Source: CAD feature listing. Evaluate the final solid. Frame: model axes, mm. Round coordinates to 2 decimals unless told otherwise and drop trailing zeros. Loops run counter-clockwise (first coordinate to the right, second up) from the corner with the lowest first, then second, coordinate; pieces in that order, holes last. Notation, with made-up numbers: (41, 54) -> (99, 54) arc R20 ccw to (99, 65) -> close; hole circle Ø3 at (47, 19.25). An arc over 180 degrees is marked (long way). Put each result on its own line as item: value. Start each with the question number.
1. Cut plane B-B (y = -195). Return the cut outline in (x, z) (3 decimals).
2. Cut plane D-D (y = 94.5). Return the cut outline in (x, z) (3 decimals), then the cut area to 3 significant figures.
3. Cut plane C-C (x = 47). Return the cut outline in (y, z) (3 decimals).
4. Contact query for flat-ended pins moving along their axis: pin 1 (3 mm diameter, centred on y = -86.5, z = 1, fed in from -X); pin 2 (3 mm diameter, centred on x = 89.5, z = 2, fed in from +Y); pin 3 (3 mm diameter, centred on x = 87.5, z = 3, fed in from -Y) (3 decimals). Output: stop coordinate, or through.
5. Cut plane A-A (x = 21). Return the cut outline in (y, z) (3 decimals), then the cut area to 3 significant figures.
6. Material intervals for L1, parallel to Y at x = 72.5, z = 4.75 (3 decimals); L2, parallel to X at y = 46, z = 2.25 (3 decimals); L3, parallel to X at y = 62, z = 3.25 (3 decimals), sorted ascending.
```python
from build123d import *

# Parameters (mm, degrees)
F1_DEPTH = 6.35
F2_R     = 3.175


with BuildPart() as f1:
    # F0 (on Top) → F1 (new body)
    with BuildSketch(Plane.XY):
        with BuildLine():
            Line((6.35, 0), (0, 0))
            Line((0, 0), (0, -19.05))
            Line((0, -19.05), (28.956, -19.05))
            ThreePointArc((28.956, -19.05), (31.201064, -18.120064), (32.131, -15.875))
            Line((32.131, -15.875), (32.131, -3.175))
            ThreePointArc((32.131, -3.175), (33.060936, -0.929936), (35.306, 0))
            Line((35.306, 0), (82.55, 0))
            ThreePointArc((82.55, 0), (84.795064, -0.929936), (85.725, -3.175))
            Line((85.725, -3.175), (85.725, -12.7))
            ThreePointArc((85.725, -12.7), (87.989524, -21.708346), (94.244716, -28.575))
            ThreePointArc((94.244716, -28.575), (115.544007, -68.2625), (94.244716, -107.95))
            ThreePointArc((94.244716, -107.95), (87.989524, -114.816654), (85.725, -123.825))
            Line((85.725, -123.825), (85.725, -133.35))
            ThreePointArc((85.725, -133.35), (84.795064, -135.595064), (82.55, -136.525))
            Line((82.55, -136.525), (3.175, -136.525))
            ThreePointArc((3.175, -136.525), (0.929936, -137.454936), (0, -139.7))
            Line((0, -139.7), (0, -171.45))
            ThreePointArc((0, -171.45), (0.929936, -173.695064), (3.175, -174.625))
            Line((3.175, -174.625), (9.525, -174.625))
            ThreePointArc((9.525, -174.625), (11.770064, -175.554936), (12.7, -177.8))
            Line((12.7, -177.8), (12.7, -184.15))
            ThreePointArc((12.7, -184.15), (11.770064, -186.395064), (9.525, -187.325))
            Line((9.525, -187.325), (0, -187.325))
            Line((0, -187.325), (0, -206.375))
            Line((0, -206.375), (28.956, -206.375))
            ThreePointArc((28.956, -206.375), (31.201064, -207.304936), (32.131, -209.55))
            Line((32.131, -209.55), (32.131, -248.9708))
            ThreePointArc((32.131, -248.9708), (33.990872, -253.460928), (38.481, -255.3208))
            Line((38.481, -255.3208), (73.025, -255.3208))
            ThreePointArc((73.025, -255.3208), (77.515128, -253.460928), (79.375, -248.9708))
            Line((79.375, -248.9708), (79.375, -190.5))
            ThreePointArc((79.375, -190.5), (80.304936, -188.254936), (82.55, -187.325))
            Line((82.55, -187.325), (104.775, -187.325))
            Line((104.775, -187.325), (104.775, -174.625))
            Line((104.775, -174.625), (111.125, -174.625))
            Line((111.125, -174.625), (111.125, -149.225))
            Line((111.125, -149.225), (104.775, -149.225))
            Line((104.775, -149.225), (104.775, -125.503588))
            ThreePointArc((104.775, -125.503588), (105.134168, -124.036716), (106.130409, -122.90172))
            ThreePointArc((106.130409, -122.90172), (134.594007, -68.2625), (106.130409, -13.62328))
            ThreePointArc((106.130409, -13.62328), (105.134168, -12.488284), (104.775, -11.021412))
            Line((104.775, -11.021412), (104.775, 12.7))
            Line((104.775, 12.7), (111.125, 12.7))
            Line((111.125, 12.7), (111.125, 38.1))
            Line((111.125, 38.1), (104.775, 38.1))
            Line((104.775, 38.1), (104.775, 50.8))
            Line((104.775, 50.8), (82.55, 50.8))
            ThreePointArc((82.55, 50.8), (80.304936, 51.729936), (79.375, 53.975))
            Line((79.375, 53.975), (79.375, 112.4458))
            ThreePointArc((79.375, 112.4458), (77.515128, 116.935928), (73.025, 118.7958))
            Line((73.025, 118.7958), (38.481, 118.7958))
            ThreePointArc((38.481, 118.7958), (33.990872, 116.935928), (32.131, 112.4458))
            Line((32.131, 112.4458), (32.131, 53.975))
            ThreePointArc((32.131, 53.975), (31.201064, 51.729936), (28.956, 50.8))
            Line((28.956, 50.8), (3.175, 50.8))
            ThreePointArc((3.175, 50.8), (0.929936, 49.870064), (0, 47.625))
            Line((0, 47.625), (0, 15.875))
            ThreePointArc((0, 15.875), (0.929936, 13.629936), (3.175, 12.7))
            Line((3.175, 12.7), (6.35, 12.7))
            ThreePointArc((6.35, 12.7), (8.595064, 11.770064), (9.525, 9.525))
            Line((9.525, 9.525), (9.525, 3.175))
            ThreePointArc((9.525, 3.175), (8.595064, 0.929936), (6.35, 0))
        make_face()
    extrude(amount=F1_DEPTH)

    # F2
    f2_edges = [f1.edges().sort_by_distance(p)[0] for p in [
        (104.775, -187.325, 3.175),
        (104.775, 50.8, 3.175),
    ]]
    fillet(f2_edges, radius=F2_R)


solid = f1.part
```
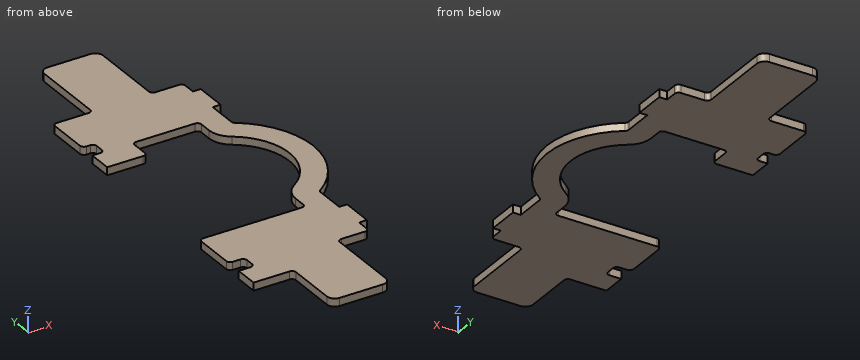
Solution:
1. outline: (0, 0) -> (79.375, 0) -> (79.375, 6.35) -> (0, 6.35) -> close
2. outline: (32.131, 0) -> (79.375, 0) -> (79.375, 6.35) -> (32.131, 6.35) -> close
2. area: 300 mm^2
3. outline: (-255.321, 0) -> (-136.525, 0) -> (-136.525, 6.35) -> (-255.321, 6.35) -> close; (0, 0) -> (118.796, 0) -> (118.796, 6.35) -> (0, 6.35) -> close
4. pin 1: stops at x = 111.26
4. pin 2: stops at y = 50.8
4. pin 3: stops at y = -187.325
5. outline: (-206.375, 0) -> (-136.525, 0) -> (-136.525, 6.35) -> (-206.375, 6.35) -> close; (-19.05, 0) -> (50.8, 0) -> (50.8, 6.35) -> (-19.05, 6.35) -> close
5. area: 887 mm^2
6. L1: y = -255.321 to -136.525, 0 to 118.796
6. L2: x = 0 to 104.775
6. L3: x = 32.131 to 79.375
